```python
from build123d import *

# Parameters (mm, degrees)
SKETCH1_R           = 1.25
BOSS_EXTRUDE1_DEPTH = 152.4


with BuildPart() as part:
    # Sketch1 → Boss-Extrude1 (new body)
    with BuildSketch(Plane(origin=(0, 0, 0), x_dir=(1, 0, 0), z_dir=(0, 1, 0))):
        with BuildLine():
            Line((-7.055036042, 2.004660127), (-6.255036042, 2.004660127))
            Line((-6.255036042, 2.004660127), (-6.255036042, 3.154660127))
            Line((-6.255036042, 3.154660127), (-3.655036042, 3.154660127))
            Line((-3.655036042, 3.154660127), (-2.655036042, 2.154660127))
            Line((-2.655036042, 2.154660127), (-2.655036042, 0.82427537))
            Line((-2.655036042, 0.82427537), (-2.355036042, 0.304660127))
            Line((-2.355036042, 0.304660127), (-2.655036042, -0.214955115))
            Line((-2.655036042, -0.214955115), (-2.655036042, -1.545339873))
            Line((-2.655036042, -1.545339873), (-3.655036042, -2.545339873))
            Line((-3.655036042, -2.545339873), (-6.255036042, -2.545339873))
            Line((-6.255036042, -2.545339873), (-6.255036042, -1.395339873))
            Line((-6.255036042, -1.395339873), (-7.055036042, -1.395339873))
            ThreePointArc((-7.055036042, -1.395339873), (-7.267168077, -1.483207838), (-7.355036042, -1.695339873))
            Line((-7.355036042, -1.695339873), (-7.355036042, -6.195339873))
            ThreePointArc((-7.355036042, -6.195339873), (-7.062142824, -6.902446654), (-6.355036042, -7.195339873))
            Line((-6.355036042, -7.195339873), (-1.855036042, -7.195339873))
            ThreePointArc((-1.855036042, -7.195339873), (-1.642904008, -7.107471907), (-1.555036042, -6.895339873))
            Line((-1.555036042, -6.895339873), (-1.555036042, -6.095339873))
            Line((-1.555036042, -6.095339873), (-2.705036042, -6.095339873))
            Line((-2.705036042, -6.095339873), (-2.705036042, -3.495339873))
            Line((-2.705036042, -3.495339873), (-1.705036042, -2.495339873))
            Line((-1.705036042, -2.495339873), (-0.374651285, -2.495339873))
            Line((-0.374651285, -2.495339873), (0.144963958, -2.195339873))
            Line((0.144963958, -2.195339873), (0.6645792, -2.495339873))
            Line((0.6645792, -2.495339873), (1.994963958, -2.495339873))
            Line((1.994963958, -2.495339873), (2.994963958, -3.495339873))
            Line((2.994963958, -3.495339873), (2.994963958, -6.095339873))
            Line((2.994963958, -6.095339873), (1.844963958, -6.095339873))
            Line((1.844963958, -6.095339873), (1.844963958, -6.895339873))
            ThreePointArc((1.844963958, -6.895339873), (1.932831923, -7.107471907), (2.144963958, -7.195339873))
            Line((2.144963958, -7.195339873), (6.644963958, -7.195339873))
            ThreePointArc((6.644963958, -7.195339873), (7.352070739, -6.902446654), (7.644963958, -6.195339873))
            Line((7.644963958, -6.195339873), (7.644963958, -1.695339873))
            ThreePointArc((7.644963958, -1.695339873), (7.557095992, -1.483207838), (7.344963958, -1.395339873))
            Line((7.344963958, -1.395339873), (6.544963958, -1.395339873))
            Line((6.544963958, -1.395339873), (6.544963958, -2.545339873))
            Line((6.544963958, -2.545339873), (3.944963958, -2.545339873))
            Line((3.944963958, -2.545339873), (2.944963958, -1.545339873))
            Line((2.944963958, -1.545339873), (2.944963958, -0.214955115))
            Line((2.944963958, -0.214955115), (2.644963958, 0.304660127))
            Line((2.644963958, 0.304660127), (2.944963958, 0.82427537))
            Line((2.944963958, 0.82427537), (2.944963958, 2.154660127))
            Line((2.944963958, 2.154660127), (3.944963958, 3.154660127))
            Line((3.944963958, 3.154660127), (6.544963958, 3.154660127))
            Line((6.544963958, 3.154660127), (6.544963958, 2.004660127))
            Line((6.544963958, 2.004660127), (7.344963958, 2.004660127))
            ThreePointArc((7.344963958, 2.004660127), (7.557095992, 2.092528093), (7.644963958, 2.304660127))
            Line((7.644963958, 2.304660127), (7.644963958, 6.804660127))
            ThreePointArc((7.644963958, 6.804660127), (7.352070739, 7.511766909), (6.644963958, 7.804660127))
            Line((6.644963958, 7.804660127), (2.144963958, 7.804660127))
            ThreePointArc((2.144963958, 7.804660127), (1.932831923, 7.716792162), (1.844963958, 7.504660127))
            Line((1.844963958, 7.504660127), (1.844963958, 6.704660127))
            Line((1.844963958, 6.704660127), (2.994963958, 6.704660127))
            Line((2.994963958, 6.704660127), (2.994963958, 4.104660127))
            Line((2.994963958, 4.104660127), (1.994963958, 3.104660127))
            Line((1.994963958, 3.104660127), (0.6645792, 3.104660127))
            Line((0.6645792, 3.104660127), (0.144963958, 2.804660127))
            Line((0.144963958, 2.804660127), (-0.374651285, 3.104660127))
            Line((-0.374651285, 3.104660127), (-1.705036042, 3.104660127))
            Line((-1.705036042, 3.104660127), (-2.705036042, 4.104660127))
            Line((-2.705036042, 4.104660127), (-2.705036042, 6.704660127))
            Line((-2.705036042, 6.704660127), (-1.555036042, 6.704660127))
            Line((-1.555036042, 6.704660127), (-1.555036042, 7.504660127))
            ThreePointArc((-1.555036042, 7.504660127), (-1.642904008, 7.716792162), (-1.855036042, 7.804660127))
            Line((-1.855036042, 7.804660127), (-6.355036042, 7.804660127))
            ThreePointArc((-6.355036042, 7.804660127), (-7.062142824, 7.511766909), (-7.355036042, 6.804660127))
            Line((-7.355036042, 6.804660127), (-7.355036042, 2.304660127))
            ThreePointArc((-7.355036042, 2.304660127), (-7.267168077, 2.092528093), (-7.055036042, 2.004660127))
        make_face()
        with Locations(Location((0.144963958, 0.304660127, 0), (0, 0, 90))):
            Circle(SKETCH1_R, mode=Mode.SUBTRACT)
    extrude(amount=BOSS_EXTRUDE1_DEPTH)


solid = part.part
```
Input: part model. Units: mm. Frame: model coordinates. A direction names the side the tool comes from. Round coordinates to 2 decimals unless told otherwise and drop trailing zeros. Answer as CSV lines item,"result".
1. Ray query, L1, parallel to X at y = 82, z = -3.75; L2, parallel to X at y = 137.5, z = 3.75; L3, parallel to Z at x = -4.5, y = 137.5. Return the intervals inside material, ascending. Write a range as [from, to].
Geometry says:
L1,"x = [-7.36, -2.35], [2.64, 7.64]"
L2,"x = [-7.36, -2.71], [2.99, 7.64]"
L3,"z = [-7.8, -3.15], [2.55, 7.2]"
2. Reachability of faces 1 (the flat face through (7.645, 75, -5)), 2 (the flat face through (-2.705, 75, 5)) from +Z, -Z, +X, -X, +Y, -Y: full face, straight path, thin tool, end or side. Return the list, or none.
Geometry says:
face 1,"+Z, -Z, +X, +Y, -Y"
face 2,"+Y, -Y"
3. Mould query, pull axis Z, two halves, no side actions, for faces 3 (the flat face through (5, 75, 2.545)), 4 (the flat face through (-4, 75, -7.805)), 5 (the flat face through (-7.355, 75, -5)). Classes: +Z half, -Z half, draft (parallel to the pull), parting line (faces both ways), or undercut.
Geometry says:
face 3,"undercut"
face 4,"-Z half"
face 5,"draft"
4. Contact query for flat-ended pins moving along their axis: P1, Ø1, axis at x = -4, z = 0.5, coming from the -Y side; P2, Ø1.1, axis at y = 41.5, z = 0.5, coming from the +X side; P3, Ø0.7, axis at x = 1, y = 92, coming from the +Z side. Output: stop coordinate, or through.
Geometry says:
P1,"passes through"
P2,"stops at x = 2.94"
P3,"stops at z = 2.5"
